```python
from build123d import *

# Parameters (mm, degrees)
SKETCH1_R           = 11.125
BOSS_EXTRUDE1_DEPTH = 10
CUT_EXTRUDE1_DEPTH  = 19.642190054
SKETCH3_W           = 17
SKETCH3_H           = 1
CUT_EXTRUDE2_DEPTH  = 19.642190054


with BuildPart() as part:
    # Sketch1 → Boss-Extrude1 (new body)
    with BuildSketch(Plane(origin=(0, 0, 0), x_dir=(1, 0, 0), z_dir=(0, 1, 0))):
        with Locations(Location((0, 0, 0), (0, 0, 270))):
            Circle(SKETCH1_R)
    extrude(amount=BOSS_EXTRUDE1_DEPTH)

    # Sketch2 → Cut-Extrude1 (cut, through all)
    with BuildSketch(Plane.XY):
        Polygon((3.469154423, 1.341962599), (7.683780529, 1.358090851), (9.777126106, 5.016128252), (7.655845577, 8.658037401), (3.441219471, 8.641909149), (1.347873894, 4.983871748), align=None)
    extrude(amount=-CUT_EXTRUDE1_DEPTH, mode=Mode.SUBTRACT)

    # Sketch3 → Cut-Extrude2 (cut, through all)
    with BuildSketch(Plane(origin=(0, 0, 0), x_dir=(1, 0, 0), z_dir=(0, 1, 0))):
        with Locations((2.926474536, 0)):
            Rectangle(SKETCH3_W, SKETCH3_H)
    extrude(amount=CUT_EXTRUDE2_DEPTH, mode=Mode.SUBTRACT)


solid = part.part
```
Geometry check sheet. Reference: the model listing, model coordinates, mm. A direction names the side the tool comes from. Give positions to 0.01 mm unless a question says otherwise; leave off trailing zeros. Loops run counter-clockwise (first coordinate to the right, second up) from the corner with the lowest first, then second, coordinate; pieces in that order, holes last. Notation, with made-up numbers: M 60,75.5 L 65,75.5 A36 ccw 65,110.5 Z; hole C 24.5,87 d3. An arc over 180 degrees is marked long. Write item = value, one per line. Start each with the question number.
1. Section check B-B, the plane y = 3. Enter the section's corners in (x, z) (3 decimals), plus the area to 3 significant figures.
2. Section check C-C, the plane x = 7.25. Enter the section's corners in (y, z).
3. Section check A-A, the plane x = 0. Enter the section's corners in (y, z) (3 decimals), plus the area to 4 significant figures.
4. Go/stop test with flat-tipped pins: P1, Ø3, axis at y = 3, z = 6.5, coming from the +X side; P2, Ø4, axis at y = 7, z = 3, coming from the -X side; P3, Ø1, axis at x = 2, y = 7.5, coming from the +Z side. Record where each tip stops, or that it passes through.
5. Section check D-D, the plane z = 0. Enter the section's corners in (x, y) (3 decimals), plus the area to 3 significant figures.
6. Thickness scan on probe 1 along Z at (x, y) = (0, 2.5) (3 decimals); probe 2 along Y at (x, z) = (7, -5.75); probe 3 along Z at (x, y) = (-1.75, 8). Record the ranges inside material, lowest first.
7. Draft check along Y on faces 1 (the face through (-5.574, 5, 0)), 2 (the face through (2.41, 6.84, -5.7)), 3 (the face through (2.394, 3.188, -5.698)), 4 (the face through (0, 0, 2)). Enter one of: +Y half, -Y half, draft (parallel to the pull), parting line (faces both ways), or undercut.
8. Tool access check on faces 5 (the face through (-8.89, 4.93, 6.69)), 6 (the face through (8.73, 6.81, -3.39)), 7 (the face through (3, 5, 0.5)). Record the directions out of +Z, -Z, +X, -X, +Y, -Y that give a thin tool (end or side, any length) a straight path to the whole face; none if there is none.
Values follow:
q1.outline = M -5.574,-0.5 L -5.574,0.5 L 11.114,0.5 A11.125 ccw long 2.503,-10.84 L 2.503,-0.5 Z; M 8.623,-7.029 A11.125 ccw 11.114,-0.5 L 8.623,-0.5 Z
q1.area = 318 mm^2
q2.outline = M 0,-8.44 L 1.36,-8.44 L 1.36,-0.5 L 0,-0.5 Z; M 0,0.5 L 10,0.5 L 10,8.44 L 0,8.44 Z; M 8.66,-8.44 L 10,-8.44 L 10,-0.5 L 8.66,-0.5 Z
q3.outline = M 0,-11.125 L 10,-11.125 L 10,-0.5 L 0,-0.5 Z; M 0,0.5 L 10,0.5 L 10,11.125 L 0,11.125 Z
q3.area = 212.5 mm^2
q4.P1 = 9.94
q4.P2 = -11.08
q4.P3 = 11.02
q5.outline = M -11.125,0 L -5.574,0 L -5.574,10 L -11.125,10 Z
q5.area = 55.5 mm^2
q6.probe_1 = -11.125 to -0.5, 0.5 to 11.125
q6.probe_2 = 0 to 1.36, 8.66 to 10
q6.probe_3 = -10.99 to -0.5, 0.5 to 10.99
q7.face_1 = draft
q7.face_2 = undercut
q7.face_3 = undercut
q7.face_4 = -Y half
q8.face_5 = +Y, -Y
q8.face_6 = -Z
q8.face_7 = +X, +Y, -Y
